from build123d import *

# Parameters (mm, degrees)
SKETCH1_W              = 482.6
SKETCH1_H              = 44.45
BOSS_EXTRUDE1_DEPTH    = 3.175
SKETCH4_R              = 6.3881
CUT_EXTRUDE1_DEPTH     = 4.175
SKETCH3_R              = 3.85
SKETCH3_R_2            = 3.2512
SKETCH3_R_3            = 1.5875
SKETCH3_W              = 17.7292
SKETCH3_H              = 16.51
CUT_EXTRUDE2_DEPTH     = 4.175
FILLET1_R              = 1.6002
LPATTERN1_COUNT        = 3
LPATTERN1_PITCH        = 127
FILLET1_OF_LPATTERN1_R = 1.6002


with BuildPart() as part:
    # Sketch1 → Boss-Extrude1 (new body)
    with BuildSketch(Plane.XY):
        Rectangle(SKETCH1_W, SKETCH1_H)
    extrude(amount=BOSS_EXTRUDE1_DEPTH)

    # Sketch4 → Cut-Extrude1 (cut, through all)
    with BuildSketch(Plane.XY.offset(3.175)):
        with Locations((-171.45, 0)):
            Circle(SKETCH4_R)
        with BuildLine():
            Line((-200.181081932, -5.1054), (-193.518918068, -5.1054))
            ThreePointArc((-193.518918068, -5.1054), (-196.85, 6.096), (-200.181081932, -5.1054))
        make_face()
    extrude(amount=-CUT_EXTRUDE1_DEPTH, mode=Mode.SUBTRACT)

    # Sketch3 → Cut-Extrude2 (cut, through all)
    with BuildSketch(Plane.XY.offset(3.175)):
        with Locations((-120.65, 0)):
            Circle(SKETCH3_R)
        with Locations((-139.7, 0)):
            Circle(SKETCH3_R_2)
        with Locations((-100.965, 11.303)):
            Circle(SKETCH3_R_3)
        with Locations((-89.535, -11.303)):
            Circle(SKETCH3_R_3)
        with Locations((-60.452, 11.303)):
            Circle(SKETCH3_R_3)
        with Locations((-49.022, -11.303)):
            Circle(SKETCH3_R_3)
        with Locations((-95.25, 0)):
            Rectangle(SKETCH3_W, SKETCH3_H)
        with Locations((-54.61, 0)):
            Rectangle(SKETCH3_W, SKETCH3_H)
    cut_extrude2 = extrude(amount=-CUT_EXTRUDE2_DEPTH, mode=Mode.SUBTRACT)

    # Fillet1
    fillet1_edges = [part.edges().sort_by_distance(p)[0] for p in [
        (-45.7454, 8.255, 1.5875),
        (-45.7454, -8.255, 1.5875),
        (-63.4746, -8.255, 1.5875),
        (-63.4746, 8.255, 1.5875),
        (-86.3854, 8.255, 1.5875),
        (-86.3854, -8.255, 1.5875),
        (-104.1146, -8.255, 1.5875),
        (-104.1146, 8.255, 1.5875),
    ]]
    fillet(fillet1_edges, radius=FILLET1_R)

    # LPattern1: Cut-Extrude2 ×3
    with Locations(*[(i * LPATTERN1_PITCH, 0, 0) for i in range(1, LPATTERN1_COUNT)]):
        add(cut_extrude2, mode=Mode.SUBTRACT)

    # Fillet1 of LPattern1
    fillet1_of_lpattern1_edges = [part.edges().sort_by_distance(p)[0] for p in [
        (81.2546, 8.255, 1.5875),
        (81.2546, -8.255, 1.5875),
        (63.5254, -8.255, 1.5875),
        (63.5254, 8.255, 1.5875),
        (40.6146, 8.255, 1.5875),
        (40.6146, -8.255, 1.5875),
        (22.8854, -8.255, 1.5875),
        (22.8854, 8.255, 1.5875),
        (208.2546, 8.255, 1.5875),
        (208.2546, -8.255, 1.5875),
        (190.5254, -8.255, 1.5875),
        (190.5254, 8.255, 1.5875),
        (167.6146, 8.255, 1.5875),
        (167.6146, -8.255, 1.5875),
        (149.8854, -8.255, 1.5875),
        (149.8854, 8.255, 1.5875),
    ]]
    fillet(fillet1_of_lpattern1_edges, radius=FILLET1_OF_LPATTERN1_R)


solid = part.part
Check sheet for the modelled part. Datum: model origin and axes. Units: mm. Round coordinates to 2 decimals unless told otherwise and drop trailing zeros. Order: outer loops, then holes, each group sorted by start corner. A loop starts at its lowest first (then second) coordinate and runs counter-clockwise, first axis right, second up.
Q1. Draft check along X on faces 1 (the face through (-177.83, 0.28, 1.61)), 2 (the face through (-3, 0, 0)), 3 (the face through (129.504, 0.169, 1.61)). Enter one of: pulls with the +X half, pulls with the -X half, needs draft (parallel to the pull), parting line crosses it, or undercut.
Filled sheet:
face 1: undercut
face 2: needs draft
face 3: undercut
Q2. Depth check by flat-ended pin: P1, Ø2.5, axis at x = 153.035, y = 11.303, coming from the +Z side. Enter the tip coordinate at first touch or a pass-through.
Filled sheet:
P1: passes through
Q3. Scan lines: L1, parallel to Y at x = -12.7, z = 2.15 (3 decimals); L2, parallel to Y at x = 191, z = 1.85 (3 decimals). Record each from-to range of solid material in increasing order.
Filled sheet:
L1: y = -22.225 to -3.251, 3.251 to 22.225
L2: y = -22.225 to -7.792, 7.792 to 22.225
Q4. Cross-section at A-A, the plane x = -171.45. Enter the section's corners in (y, z) (3 decimals).
Filled sheet:
outline: (-22.225, 0) - (-6.388, 0) - (-6.388, 3.175) - (-22.225, 3.175) - close; (6.388, 0) - (22.225, 0) - (22.225, 3.175) - (6.388, 3.175) - close
Q5. Cross-section at B-B, the plane z = 1.35. Give the number of separate pieces and of enclosed holes in the cut face, plus the area to 3 significant figures.
Filled sheet:
separate pieces: 1
enclosed holes: 26
area: 19,100 mm2
